The model under review builds one solid part; all positions refer to its coordinate system, in mm. Face numbers are marked on the shaded views. Give positions to 0.01 mm unless a question says otherwise; leave off trailing zeros. Order: outer loops, then holes, each group sorted by start corner. A loop starts at its lowest first (then second) coordinate and runs counter-clockwise, first axis right, second up. Notation, with made-up numbers: (13.25, -24) - (52.25, -24) arc R27 ccw to (52.25, -8) - close; hole circle Ø4 at (-24.75, -11). An arc over 180 degrees is marked (long way). Use CSV: the item, a comma, the result in double quotes.
```python
from build123d import *

# Parameters (mm, degrees)
SKETCH1_W           = 600
SKETCH1_H           = 260
BOSS_EXTRUDE1_DEPTH = 100
SHELL1_T            = 2
SKETCH2_W           = 92.440689116
SKETCH2_H           = 25.153929011
SKETCH2_W_2         = 82.440689116
SKETCH2_H_2         = 15.153929011
BOSS_EXTRUDE2_DEPTH = 10
SKETCH2_3_W         = 82.440689116
SKETCH2_3_H         = 15.153929011
SKETCH2_3_W_2       = 9.01524931
SKETCH2_3_H_2       = 10.647439476
BOSS_EXTRUDE3_DEPTH = 6
FILLET1_R           = 10


with BuildPart() as part:
    # Sketch1 → Boss-Extrude1 (new body)
    with BuildSketch(Plane(origin=(0, 0, 0), x_dir=(1, 0, 0), z_dir=(0, 1, 0))):
        Rectangle(SKETCH1_W, SKETCH1_H)
    extrude(amount=BOSS_EXTRUDE1_DEPTH)

    # Shell1 (no face opened: a closed hollow body)
    add(offset(amount=-SHELL1_T, mode=Mode.PRIVATE), mode=Mode.SUBTRACT)

    # Sketch2 → Boss-Extrude2 (add)
    with BuildSketch(Plane.XY.offset(130)):
        with Locations((0, 46.226910649)):
            Rectangle(SKETCH2_W, SKETCH2_H)
        with Locations((0, 46.226910649)):
            Rectangle(SKETCH2_W_2, SKETCH2_H_2, mode=Mode.SUBTRACT)
    extrude(amount=BOSS_EXTRUDE2_DEPTH)

    # Sketch2<3> → Boss-Extrude3 (add)
    with BuildSketch(Plane.XY.offset(130)):
        with Locations((0, 46.226910649)):
            Rectangle(SKETCH2_3_W, SKETCH2_3_H)
        with Locations((35.85201026, 46.226910648)):
            Rectangle(SKETCH2_3_W_2, SKETCH2_3_H_2, mode=Mode.SUBTRACT)
        with Locations((25.85201026, 46.226910648)):
            Rectangle(SKETCH2_3_W_2, SKETCH2_3_H_2, mode=Mode.SUBTRACT)
        with Locations((15.85201026, 46.226910648)):
            Rectangle(SKETCH2_3_W_2, SKETCH2_3_H_2, mode=Mode.SUBTRACT)
        with Locations((5.85201026, 46.226910648)):
            Rectangle(SKETCH2_3_W_2, SKETCH2_3_H_2, mode=Mode.SUBTRACT)
        with Locations((-4.14798974, 46.226910648)):
            Rectangle(SKETCH2_3_W_2, SKETCH2_3_H_2, mode=Mode.SUBTRACT)
        with Locations((-14.14798974, 46.226910648)):
            Rectangle(SKETCH2_3_W_2, SKETCH2_3_H_2, mode=Mode.SUBTRACT)
        with Locations((-24.14798974, 46.226910648)):
            Rectangle(SKETCH2_3_W_2, SKETCH2_3_H_2, mode=Mode.SUBTRACT)
        with Locations((-34.14798974, 46.226910648)):
            Rectangle(SKETCH2_3_W_2, SKETCH2_3_H_2, mode=Mode.SUBTRACT)
    extrude(amount=BOSS_EXTRUDE3_DEPTH)

    # Fillet1
    fillet1_edges = [part.edges().sort_by_distance(p)[0] for p in [
        (46.220344558, 46.226910648, 130),
        (0, 58.803875154, 130),
        (-46.220344558, 46.226910648, 130),
        (0, 33.649946143, 130),
    ]]
    fillet(fillet1_edges, radius=FILLET1_R - 0.0001)  # a hair under: the kernel refuses the full size


solid = part.part
```
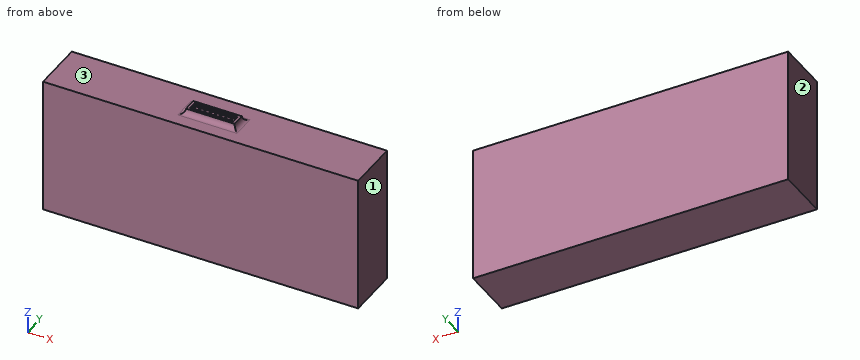
Item 1: Take a section at B-B, the plane x = -102. Give the boundary of the cut face in (y, z).
Results list:
outline,"(0, -130) - (100, -130) - (100, 130) - (0, 130) - close; hole (2, -128) - (98, -128) - (98, 128) - (2, 128) - close"
Item 2: Wall thickness on L1, parallel to Z at x = 198, y = 41; L2, parallel to Y at x = -267, z = -86; L3, parallel to X at y = 63, z = -1: over which ranges is each line inside the solid? List them lowest first.
Results list:
L1,"z = -130 to -128, 128 to 130"
L2,"y = 0 to 2, 98 to 100"
L3,"x = -300 to -298, 298 to 300"
Item 3: Clearance check with flat-ended pins moving along their axes: pin 1 (4.5 mm diameter, centred on y = 48.5, z = 138, fed in from -X); pin 2 (3 mm diameter, centred on y = 44.5, z = 138.5, fed in from +X); pin 3 (1.8 mm diameter, centred on x = -5.5, z = 132.5, fed in from -Y). State where each tip first meets the part, or that it passes through.
Results list:
pin 1,"stops at x = -47.17"
pin 2,"stops at x = 46.68"
pin 3,"stops at y = 29.08"
Item 4: Take a section at A-A, the plane y = 17. Give the boundary of the cut face in (x, z), and give its area (3 significant figures).
Results list:
outline,"(-300, -130) - (300, -130) - (300, 130) - (-300, 130) - close; hole (-298, -128) - (298, -128) - (298, 128) - (-298, 128) - close"
area,"3,420 mm2"
Item 5: Mouldability with a two-part tool opening along X and no side actions: class the marked faces 1, 2 and 3 as pulls with the +X half, pulls with the -X half, needs draft (parallel to the pull), parting line crosses it, or undercut.
Results list:
face 1,"pulls with the +X half"
face 2,"pulls with the -X half"
face 3,"needs draft"
